from build123d import *

# Parameters (mm, degrees)
F1_DEPTH = 0.15


with BuildPart() as f1:
    # F0 (on Top) → F1 (new body)
    with BuildSketch(Plane.XY):
        with BuildLine():
            Line((12, 0.08), (0.632456, 0.15))
            ThreePointArc((0.632456, 0.15), (0.005149, 0.64998), (-0.63, 0.16))
            Line((-0.63, 0.16), (-3, 0.21))
            Line((-3, 0.21), (-3, 0))
            Line((-3, 0), (-3, -0.21))
            Line((-3, -0.21), (-0.63, -0.16))
            ThreePointArc((-0.63, -0.16), (0.005149, -0.64998), (0.632456, -0.15))
            Line((0.632456, -0.15), (12, -0.08))
            Line((12, -0.08), (12, 0))
            Line((12, 0), (12, 0.08))
        make_face()
    extrude(amount=F1_DEPTH)


solid = f1.part
Could you check a few things on this model? Use its own coordinates, in mm. Round coordinates to 2 decimals unless told otherwise and drop trailing zeros. Write each loop counter-clockwise with the first axis right and the second up, starting at its lowest first coordinate (ties: lowest second). Pieces come first, ordered by that corner, then holes. Notation, with made-up numbers: (37.25, -31.75) - (93.25, -31.75) arc R32 cw to (93.25, 6.25) - close; hole circle Ø10 at (85, 75.5). An arc over 180 degrees is marked (long way). Put each result on its own line as item: value. Start each with the question number.
(1) I want a section at C-C, the plane y = 0.5. Please give me the cut outline in (x, z), plus the area to 3 significant figures.
(2) I want a section at A-A, the plane z = 0.1. Please give me the cut outline in (x, y), plus the area to 3 significant figures.
(3) I need wall thicknesses on probe 1 along X at (y, z) = (0.55, 0.1); probe 2 along X at (y, z) = (-0.3, 0.1); probe 3 along Y at (x, z) = (7, 0.1). Which ranges of each line are inside material? Lowest first, please.
(4) I want a section at B-B, the plane x = -1.5. Please give me the cut outline in (y, z), plus the area to 3 significant figures.
Here are the results:
1. outline: (-0.42, 0) - (0.42, 0) - (0.42, 0.15) - (-0.42, 0.15) - close
1. area: 0.125 mm^2
2. outline: (-3, -0.21) - (-0.63, -0.16) arc R0.65 ccw to (0.63, -0.15) - (12, -0.08) - (12, 0.08) - (0.63, 0.15) arc R0.65 ccw to (-0.63, 0.16) - (-3, 0.21) - close
2. area: 4.81 mm^2
3. probe 1: x = -0.35 to 0.35
3. probe 2: x = -0.58 to 0.58
3. probe 3: y = -0.11 to 0.11
4. outline: (-0.18, 0) - (0.18, 0) - (0.18, 0.15) - (-0.18, 0.15) - close
4. area: 0.0535 mm^2
